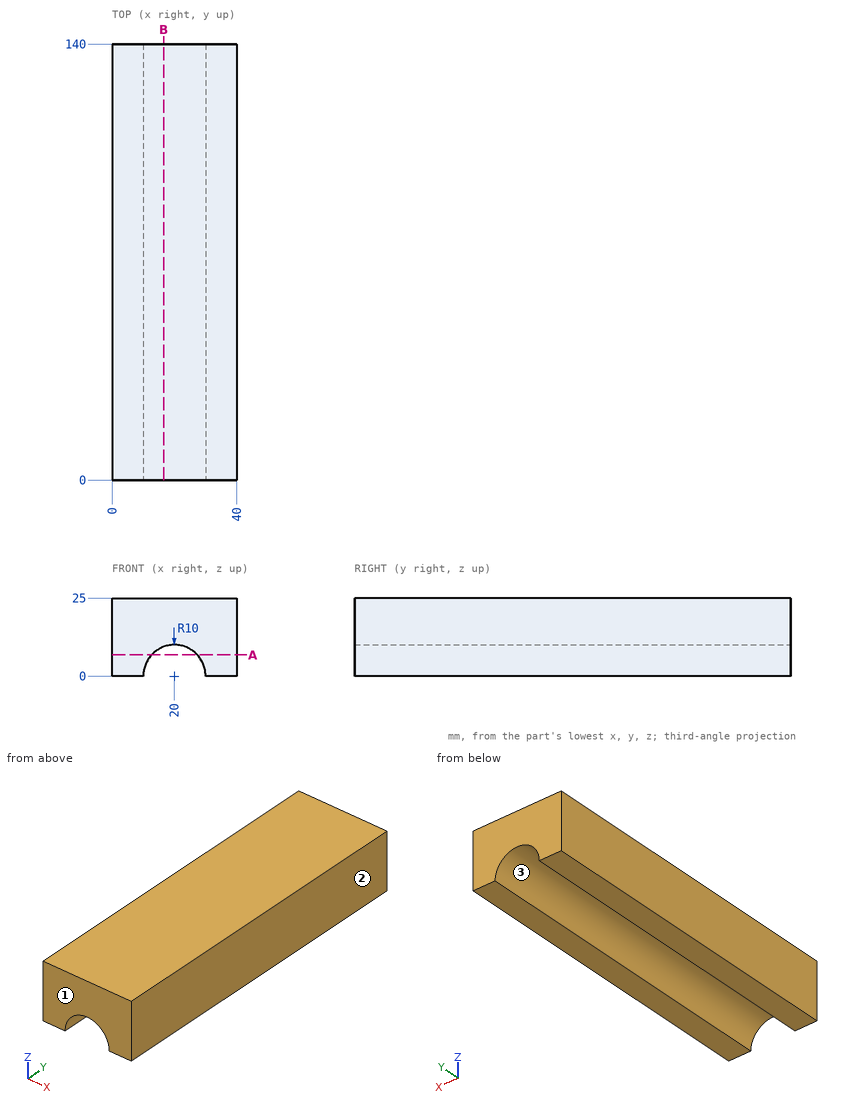
Answer from the drawing. Dimensions are ordinates in mm from the lowest x, y and z of the part. Coordinates: 2 decimals unless noted, no trailing zeros. Loops run counter-clockwise (first coordinate to the right, second up) from the corner with the lowest first, then second, coordinate; pieces in that order, holes last. Notation, with made-up numbers: (-7.75, -28) - (24.25, -28) arc R32 ccw to (24.25, 2) - close; hole circle Ø5 at (-17.5, 79). An arc over 180 degrees is marked (long way). Answer in a Markdown table with one row per item.
1. Determine the mould class of the marked faces 1, 2 and 3 for opening direction X: +X half, -X half, draft (parallel to the pull), parting line (faces both ways), or undercut.
Conclusion:
| item | result |
|---|---|
| face 1 | draft |
| face 2 | +X half |
| face 3 | undercut |
2. Given pin 1 (3 mm diameter, centred on x = 27, y = 120.5, fed in from -Z), flat-ended and moving along its own axis, determine where the tip first touches the part or whether it passes through.
Conclusion:
| item | result |
|---|---|
| pin 1 | stops at z = 5.27 |
3. Find section B-B, the plane x = 16.5. Write down the section's boundary in (y, z).
Conclusion:
| item | result |
|---|---|
| outline | (0, 9.37) - (140, 9.37) - (140, 25) - (0, 25) - close |
4. Straight lines are drawn through the part: line 1 (X direction, y = 43, z = 8); line 2 (X direction, y = 21.5, z = 7.75); line 3 (Z direction, x = 28.5, y = 113). For each, find the intervals that lie inside material, in ascending order.
Conclusion:
| item | result |
|---|---|
| line 1 | x = 0 to 14, 26 to 40 |
| line 2 | x = 0 to 13.68, 26.32 to 40 |
| line 3 | z = 5.27 to 25 |
5. Find section A-A, the plane z = 6.75. Write down the section's boundary in (x, y), then the cut area to 3 significant figures.
Conclusion:
| item | result |
|---|---|
| outline | (0, 0) - (12.62, 0) - (12.62, 140) - (0, 140) - close; (27.38, 0) - (40, 0) - (40, 140) - (27.38, 140) - close |
| area | 3,530 mm² |
